```python
from build123d import *


with BuildPart() as part:
    # Sketch 1 → Revolve 1 (revolve)
    with BuildSketch(Plane.XY, mode=Mode.PRIVATE) as revolve_1_sk:
        with BuildLine():
            Line((0, 14), (0, 12.8))
            Line((0, 12.8), (0.55, 12.8))
            Line((0.55, 12.8), (0.55, 9.3))
            Line((0.55, 9.3), (0, 9.3))
            Line((0, 9.3), (0, 7.8))
            ThreePointArc((0, 7.8), (0.087867966, 7.587867966), (0.3, 7.5))
            Line((0.3, 7.5), (6.7, 7.5))
            ThreePointArc((6.7, 7.5), (6.912132034, 7.587867966), (7, 7.8))
            Line((7, 7.8), (7, 9.3))
            Line((7, 9.3), (6.45, 9.3))
            Line((6.45, 9.3), (6.45, 12.8))
            Line((6.45, 12.8), (7, 12.8))
            Line((7, 12.8), (7, 13.7))
            ThreePointArc((7, 13.7), (6.912132034, 13.912132034), (6.7, 14))
            Line((6.7, 14), (0, 14))
        make_face()
    revolve(revolve_1_sk.sketch.rotate(Axis((7, 0, 0), (-1, 0, 0)), 270), axis=Axis((7, 0, 0), (-1, 0, 0)))


solid = part.part
```
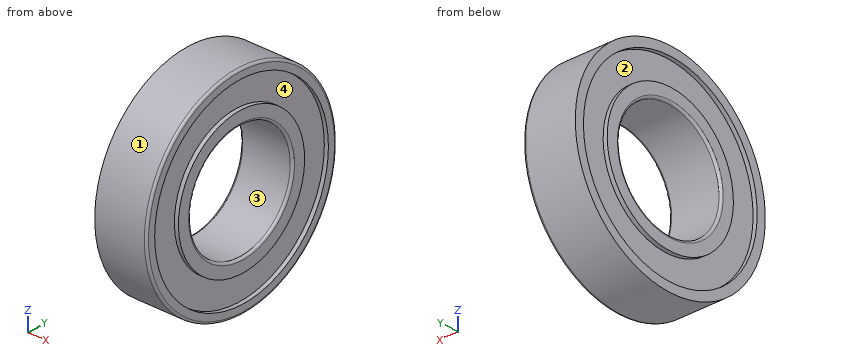
For this review, take the finished solid that the model builds, in its own axes (mm). Face numbers are marked on the shaded views. A direction names the side the tool comes from. Round coordinates to 2 decimals unless told otherwise and drop trailing zeros. Loops run counter-clockwise (first coordinate to the right, second up) from the corner with the lowest first, then second, coordinate; pieces in that order, holes last.
(1) Tool access review of the marked faces 3 and 4: name each direction out of +Z, -Z, +X, -X, +Y, -Y from which nothing blocks a thin tool from reaching the whole face with its end or side.
Returned:
face 3: +X, -X
face 4: +X
(2) Clearance check with flat-ended pins moving along their axes: P1, Ø1, axis at x = 4.5, z = 0.5, coming from the -Y side; P2, Ø2, axis at x = 1, z = -3, coming from the -Y side; P3, Ø9, axis at y = 0, z = 0, coming from the +X side. State where each tip first meets the part, or that it passes through.
Returned:
P1: stops at y = -14
P2: stops at y = -13.86
P3: passes through
(3) Mouldability with a two-part tool opening along Z and no side actions: class the marked faces 1 and 2 as released by +Z, released by -Z, zero draft, split by the parting line, or undercut.
Returned:
face 1: split by the parting line
face 2: undercut
(4) Wall thickness on line 1 along Y through (x, z) = (6.85, 0); line 2 along Z through (x, y) = (2.5, -1); line 3 along X through (y, z) = (-6.5, 7): over which ranges is each line inside the solid? List them lowest first.
Returned:
line 1: y = -13.96 to -12.8, -9.3 to -7.54, 7.54 to 9.3, 12.8 to 13.96
line 2: z = -13.96 to -7.43, 7.43 to 13.96
line 3: x = 0.55 to 6.45
(5) We need section C-C (x = 3.25). Give the boundary of the cut face in (y, z).
Returned:
outline: circle Ø28 at (0, 0); hole circle Ø15 at (0, 0)
